Could you check a few things on this model? Use its own coordinates, in mm. Coordinates: 2 decimals unless noted, no trailing zeros. Put each result on its own line as item: value. Start each with the question number.
```python
from build123d import *

# Parameters (mm, degrees)
ESQUISSE1_W             = 40
ESQUISSE1_H             = 80
ESQUISSE1_R             = 3
BOSS_EXTRU_1_DEPTH      = 5
ESQUISSE2_R             = 2.5
ESQUISSE2_W             = 30
ESQUISSE2_H             = 30
ESQUISSE2_W_2           = 25
ESQUISSE2_H_2           = 10
ENL_V_MAT_EXTRU_1_DEPTH = 209.386659842
ESQUISSE4_W             = 20
ESQUISSE4_H             = 20
ENL_V_MAT_EXTRU_2_DEPTH = 10


with BuildPart() as part:
    # Esquisse1 → Boss.-Extru.1 (new body)
    # profile 1 of 7: a face of its own
    with BuildSketch(Plane(origin=(0, 0, 0), x_dir=(1, 0, 0), z_dir=(0, 1, 0))):
        with BuildLine():
            ThreePointArc((4.38e-07, -150), (-90.829510449, -119.373363996), (-144.568322948, -40))
            Line((-144.568322948, -40), (-144.568322948, -150))
            Line((-144.568322948, -150), (4.38e-07, -150))
        make_face()
    # profile 2 of 7: a face of its own
    with BuildSketch(Plane(origin=(0, 0, 0), x_dir=(1, 0, 0), z_dir=(0, 1, 0))):
        with BuildLine():
            ThreePointArc((144.568322948, -40), (90.829510797, -119.373363731), (4.38e-07, -150))
            Line((4.38e-07, -150), (144.568322948, -150))
            Line((144.568322948, -150), (144.568322948, -40))
        make_face()
    # profile 3 of 7: a face of its own
    with BuildSketch(Plane(origin=(0, 0, 0), x_dir=(1, 0, 0), z_dir=(0, 1, 0))):
        with Locations((124.568322948, 0)):
            Rectangle(ESQUISSE1_W, ESQUISSE1_H)
    # profile 4 of 7: a face of its own
    with BuildSketch(Plane(origin=(0, 0, 0), x_dir=(1, 0, 0), z_dir=(0, 1, 0))):
        with BuildLine():
            ThreePointArc((2.28e-07, 150), (-90.829510532, 119.373363932), (-144.568322948, 40))
            Line((-144.568322948, 40), (-104.568322948, 40))
            Line((-104.568322948, 40), (-104.568322948, -40))
            Line((-104.568322948, -40), (-144.568322948, -40))
            ThreePointArc((-144.568322948, -40), (-90.829510449, -119.373363996), (4.38e-07, -150))
            ThreePointArc((4.38e-07, -150), (90.829510797, -119.373363731), (144.568322948, -40))
            Line((144.568322948, -40), (104.568322948, -40))
            Line((104.568322948, -40), (104.568322948, 40))
            Line((104.568322948, 40), (144.568322948, 40))
            ThreePointArc((144.568322948, 40), (90.829510714, 119.373363794), (2.28e-07, 150))
        make_face()
        with Locations(Location((-124.568322948, -60, 0), (0, 0, 270))):
            Circle(ESQUISSE1_R, mode=Mode.SUBTRACT)
        with Locations(Location((124.568322948, -60, 0), (0, 0, 270))):
            Circle(ESQUISSE1_R, mode=Mode.SUBTRACT)
        with Locations(Location((-124.568322948, 60, 0), (0, 0, 270))):
            Circle(ESQUISSE1_R, mode=Mode.SUBTRACT)
        with Locations(Location((124.568322948, 60, 0), (0, 0, 270))):
            Circle(ESQUISSE1_R, mode=Mode.SUBTRACT)
    # profile 5 of 7: a face of its own
    with BuildSketch(Plane(origin=(0, 0, 0), x_dir=(1, 0, 0), z_dir=(0, 1, 0))):
        with Locations((-124.568322948, 0)):
            Rectangle(ESQUISSE1_W, ESQUISSE1_H)
    # profile 6 of 7: a face of its own
    with BuildSketch(Plane(origin=(0, 0, 0), x_dir=(1, 0, 0), z_dir=(0, 1, 0))):
        with BuildLine():
            Line((-144.568322948, 150), (-144.568322948, 40))
            ThreePointArc((-144.568322948, 40), (-90.829510532, 119.373363932), (2.28e-07, 150))
            Line((2.28e-07, 150), (-144.568322948, 150))
        make_face()
    # profile 7 of 7: a face of its own
    with BuildSketch(Plane(origin=(0, 0, 0), x_dir=(1, 0, 0), z_dir=(0, 1, 0))):
        with BuildLine():
            Line((144.568322948, 150), (2.28e-07, 150))
            ThreePointArc((2.28e-07, 150), (90.829510714, 119.373363794), (144.568322948, 40))
            Line((144.568322948, 40), (144.568322948, 150))
        make_face()
    extrude(amount=BOSS_EXTRU_1_DEPTH)

    # Esquisse2 → Enlèv. mat.-Extru.1 (cut, through all)
    with BuildSketch(Plane(origin=(0, 5, 0), x_dir=(1, 0, 0), z_dir=(0, 1, 0))):
        with Locations(Location((25, -45, 0), (0, 0, 270))):
            Circle(ESQUISSE2_R)
        with Locations(Location((25, -65, 0), (0, 0, 270))):
            Circle(ESQUISSE2_R)
        with Locations(Location((-25, -45, 0), (0, 0, 270))):
            Circle(ESQUISSE2_R)
        with Locations(Location((-25, -65, 0), (0, 0, 270))):
            Circle(ESQUISSE2_R)
        with BuildLine():
            Line((23, -25), (-23, -25))
            ThreePointArc((-23, -25), (-24.414213562, -24.414213562), (-25, -23))
            Line((-25, -23), (-25, 23))
            ThreePointArc((-25, 23), (-24.414213562, 24.414213562), (-23, 25))
            Line((-23, 25), (23, 25))
            ThreePointArc((23, 25), (24.414213562, 24.414213562), (25, 23))
            Line((25, 23), (25, -23))
            ThreePointArc((25, -23), (24.414213562, -24.414213562), (23, -25))
        make_face()
        with Locations((0, -58)):
            Rectangle(ESQUISSE2_W, ESQUISSE2_H)
        with Locations((0, -35)):
            Rectangle(ESQUISSE2_W_2, ESQUISSE2_H_2)
    extrude(amount=-ENL_V_MAT_EXTRU_1_DEPTH, mode=Mode.SUBTRACT)

    # Esquisse4 → Enlèv. mat.-Extru.2 (cut)
    with BuildSketch(Plane(origin=(0, 5, 0), x_dir=(1, 0, 0), z_dir=(0, 1, 0))):
        with Locations((-134.568322948, 140)):
            Rectangle(ESQUISSE4_W, ESQUISSE4_H)
        with Locations((134.568322948, 140)):
            Rectangle(ESQUISSE4_W, ESQUISSE4_H)
        with Locations((134.568322948, -140)):
            Rectangle(ESQUISSE4_W, ESQUISSE4_H)
        with Locations((-134.568322948, -140)):
            Rectangle(ESQUISSE4_W, ESQUISSE4_H)
    extrude(amount=-ENL_V_MAT_EXTRU_2_DEPTH, mode=Mode.SUBTRACT)


solid = part.part
```
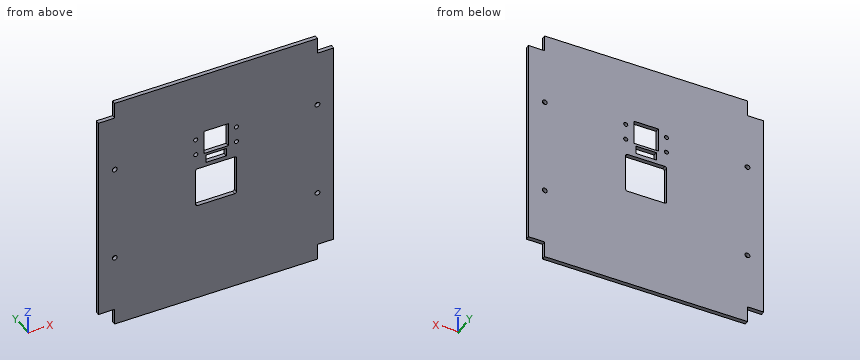
Item 1: I need wall thicknesses on probe 1 along Z at (x, y) = (-9, 1.3); probe 2 along X at (y, z) = (2.5, 60); probe 3 along X at (y, z) = (4, 45). Which ranges of each line are inside material? Lowest first, please.
Item 2: For pin 1 Ø4.5 at (x, z) = (25, 65) entering from +Y; pin 2 Ø1.5 at (x, z) = (41, 51.5) entering from -Y; pin 3 Ø2.5 at (y, z) = (1.5, -136) entering from +X; pin 4 Ø1.5 at (x, y) = (135.5, 3) entering from -Z, each with a flat end and sliding along its axis, tell me the tip position at first contact or that it passes through.
Item 3: If we section it at A-A on y = 3.9: State how many separate pieces and enclosed holes the cut face has, then the cut area to 3 significant figures.
Geometry check:
1. probe 1: z = -150 to -25, 25 to 30, 40 to 43, 73 to 150
1. probe 2: x = -144.57 to -127.57, -121.57 to -15, 15 to 121.57, 127.57 to 144.57
1. probe 3: x = -144.57 to -27.5, -22.5 to -15, 15 to 22.5, 27.5 to 144.57
2. pin 1: passes through
2. pin 2: stops at y = 0
2. pin 3: stops at x = 124.57
2. pin 4: stops at z = -130
3. separate pieces: 1
3. enclosed holes: 11
3. area: 81,300 mm²
